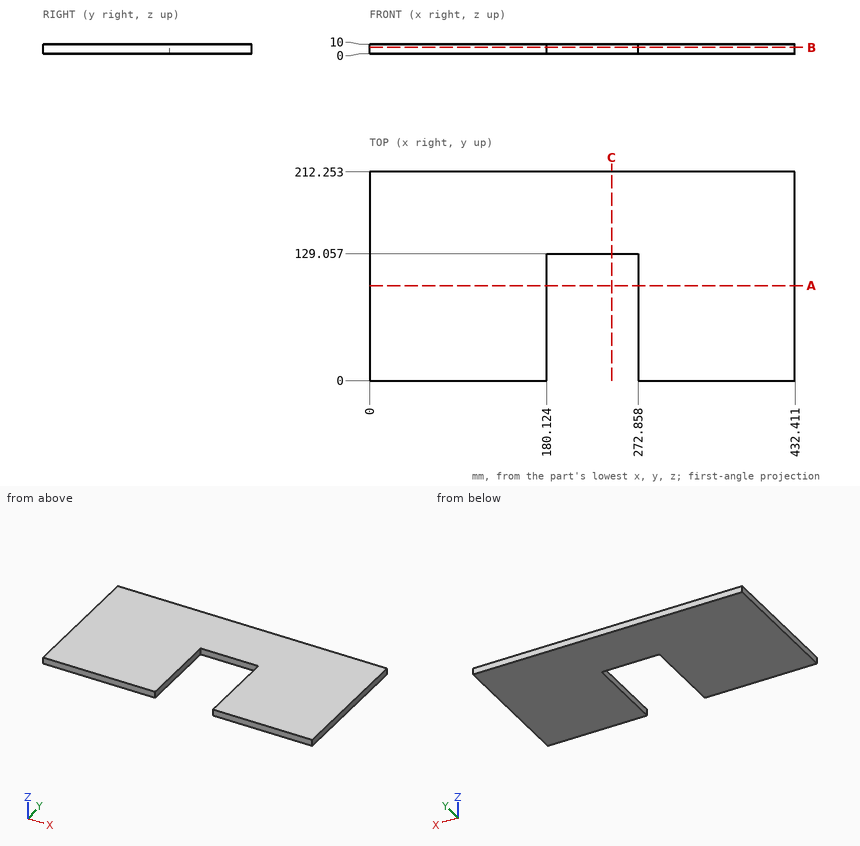
The figure shows three views and two pictorial views of one solid part (mm, origin at its lowest corner). Answer the questions. Coordinates: 2 decimals unless noted, no trailing zeros. Order: outer loops, then holes, each group sorted by start corner. A loop starts at its lowest first (then second) coordinate and runs counter-clockwise, first axis right, second up. Notation, with made-up numbers: (13.5, 73) - (55.5, 73) arc R24 ccw to (55.5, 99) - close; hole circle Ø1 at (-6, 36). An arc over 180 degrees is marked (long way). Answer as a JSON object with one key per item and string values.
1. Find section A-A on y = 96.5. Determine the outline of the cut face in (x, z), plus the area to 3 significant figures.
Output values:
{"outline": "(0, 0) - (180.12, 0) - (180.12, 10) - (0, 10) - close; (272.86, 0) - (432.41, 0) - (432.41, 10) - (272.86, 10) - close", "area": "3,400 mm²"}
2. Each of these flat-tipped pins is pushed along its axis until it touches: P1, Ø3, axis at x = 319, y = 24, coming from the -Z side; P2, Ø3, axis at x = 215, z = 5, coming from the -Y side. Where does it stop, or does it pass through?
Output values:
{"P1": "stops at z = 0", "P2": "stops at y = 129.06"}
3. Find section C-C on x = 246. Determine the outline of the cut face in (y, z), plus the area to 3 significant figures.
Output values:
{"outline": "(129.06, 0) - (212.25, 0) - (212.25, 10) - (129.06, 10) - close", "area": "832 mm²"}
4. Consider line 1 (X direction, y = 58.5, z = 4.75); line 2 (Y direction, x = 259, z = 6). Determine where each line is inside the solid, lowest interval first.
Output values:
{"line 1": "x = 0 to 180.12, 272.86 to 432.41", "line 2": "y = 129.06 to 212.25"}
5. Find section B-B on z = 6.5. Determine the outline of the cut face in (x, y).
Output values:
{"outline": "(0, 0) - (180.12, 0) - (180.12, 129.06) - (272.86, 129.06) - (272.86, 0) - (432.41, 0) - (432.41, 212.25) - (0, 212.25) - close"}
